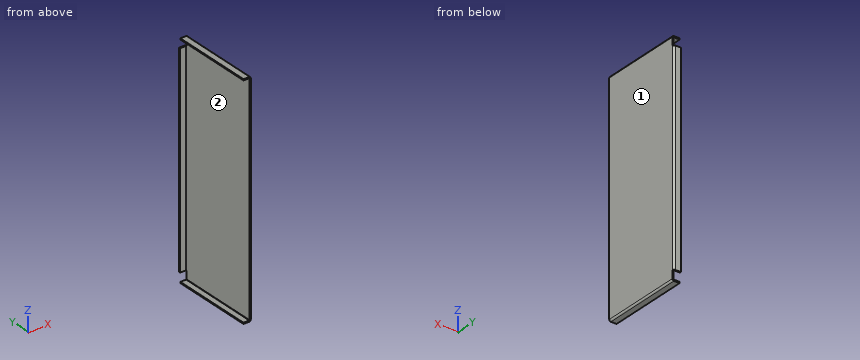
```python
from build123d import *

# Parameters (mm, degrees)
SKETCH1_W               = 575.31
SKETCH1_H               = 214.9475
BASE_FLANGE1_DEPTH      = 3.175
EDGE_FLANGE1_DEPTH      = 214.9475
EDGE_FLANGE1_BEND_DEPTH = 214.9475
EDGE_FLANGE2_DEPTH      = 537.75


# Sheet-metal steps are written as plain solids
with BuildPart() as part:
    # Sketch1 → Base-Flange1 (new body)
    with BuildSketch(Plane(origin=(0, 0, 0), x_dir=(0, 0, -1), z_dir=(1, 0, 0))):
        Rectangle(SKETCH1_W, SKETCH1_H)
    extrude(amount=-BASE_FLANGE1_DEPTH)

    # Edge-Flange1 section (across the edge) → Edge-Flange1 (add)
    with BuildSketch(Plane(origin=(-3.175, 107.47375, -290.195), x_dir=(0, 0, 1), z_dir=(0, -1, 0))):
        with BuildLine():
            Line((-3.175, 1), (-3.175, 15.875))
            Line((-3.175, 15.875), (0, 15.875))
            Line((0, 15.875), (0, 1))
            ThreePointArc((0, 1), (0.292893219, 0.292893219), (1, 0))
            Line((1, 0), (2.54, 0))
            Line((2.54, 0), (2.54, -3.175))
            Line((2.54, -3.175), (1, -3.175))
            ThreePointArc((1, -3.175), (-1.952170811, -1.952170811), (-3.175, 1))
        make_face()
    extrude(amount=EDGE_FLANGE1_DEPTH)

    # Edge-Flange1 section 2 (across the edge) → Edge-Flange1 bend (add)
    with BuildSketch(Plane(origin=(-3.175, -107.47375, 290.195), x_dir=(0, 0, -1), z_dir=(0, 1, 0))):
        with BuildLine():
            Line((-3.175, 1), (-3.175, 15.875))
            Line((-3.175, 15.875), (0, 15.875))
            Line((0, 15.875), (0, 1))
            ThreePointArc((0, 1), (0.292893219, 0.292893219), (1, 0))
            Line((1, 0), (2.54, 0))
            Line((2.54, 0), (2.54, -3.175))
            Line((2.54, -3.175), (1, -3.175))
            ThreePointArc((1, -3.175), (-1.952170811, -1.952170811), (-3.175, 1))
        make_face()
    extrude(amount=EDGE_FLANGE1_BEND_DEPTH)

    # Edge-Flange2 section (across the edge) → Edge-Flange2 (add)
    with BuildSketch(Plane(origin=(-3.175, 108.74375, 268.875), x_dir=(0, -1, 0), z_dir=(0, 0, -1))):
        with BuildLine():
            Line((-3.175, 1), (-3.175, 15.326869713))
            Line((-3.175, 15.326869713), (0, 15.326869713))
            Line((0, 15.326869713), (0, 1))
            ThreePointArc((0, 1), (0.292893219, 0.292893219), (1, 0))
            Line((1, 0), (1.27, 0))
            Line((1.27, 0), (1.27, -3.175))
            Line((1.27, -3.175), (1, -3.175))
            ThreePointArc((1, -3.175), (-1.952170811, -1.952170811), (-3.175, 1))
        make_face()
    extrude(amount=EDGE_FLANGE2_DEPTH)


solid = part.part
```
Source: CAD feature listing. Evaluate the final solid. Frame: model axes, mm. Face numbers are marked on the shaded views. Give positions to 0.01 mm unless a question says otherwise; leave off trailing zeros. Loops run counter-clockwise (first coordinate to the right, second up) from the corner with the lowest first, then second, coordinate; pieces in that order, holes last. Notation, with made-up numbers: M 63,77.5 L 102,77.5 A17 cw 102,90.5 Z; hole C 49.5,52 d9. An arc over 180 degrees is marked long. Put each result on its own line as item: value.
Q1. Mould query, pull axis Z, two halves, no side actions, for the marked faces 1 and 2. Classes: released by +Z, released by -Z, zero draft, split by the parting line, or undercut.
Response values:
face 1: zero draft
face 2: undercut
Q2. Section B-B (z = 181). Return the cut outline in (x, y) (3 decimals), and give its area (3 significant figures).
Response values:
outline: M -18.502,108.744 L -4.175,108.744 A1 cw -3.175,107.744 L -3.175,-107.474 L 0,-107.474 L 0,107.744 A4.175 ccw -4.175,111.919 L -18.502,111.919 Z
area: 742 mm²
Q3. Pin query (flat end, axial travel): P1, Ø3.5, axis at x = -8, y = 109.5, coming from the -Z side (3 decimals); P2, Ø1.6, axis at y = 110.5, z = -47.5, coming from the -X side; P3, Ø6, axis at y = 14, z = -194, coming from the -X side (3 decimals). Return the tip coordinate at first contact, or that it passes through.
Response values:
P1: stops at z = -268.875
P2: stops at x = -18.5
P3: stops at x = -3.175
Q4. Line query: probe 1 along Z at (x, y) = (-9.5, 91) (3 decimals); probe 2 along Y at (x, z) = (-7.75, 248.5); probe 3 along X at (y, z) = (-66, 112) (3 decimals). Output: solid intervals per line, ascending. Write a range as [from, to].
Response values:
probe 1: z = [-293.37, -290.195], [290.195, 293.37]
probe 2: y = [108.74, 111.92]
probe 3: x = [-3.175, 0]
Q5. Section A-A (x = -9.75). Return the cut outline in (y, z) (3 decimals).
Response values:
outline: M -107.474,-293.37 L 107.474,-293.37 L 107.474,-290.195 L -107.474,-290.195 Z; M -107.474,290.195 L 107.474,290.195 L 107.474,293.37 L -107.474,293.37 Z; M 108.744,-268.875 L 111.919,-268.875 L 111.919,268.875 L 108.744,268.875 Z
Q6. Section C-C (y = -78.5). Return the cut outline in (x, z) (3 decimals), and give its area (3 significant figures).
Response values:
outline: M -19.05,-293.37 L -4.175,-293.37 A4.175 ccw 0,-289.195 L 0,289.195 A4.175 ccw -4.175,293.37 L -19.05,293.37 L -19.05,290.195 L -4.175,290.195 A1 cw -3.175,289.195 L -3.175,-289.195 A1 cw -4.175,-290.195 L -19.05,-290.195 Z
area: 1,960 mm²
